Geometry check sheet. Reference: the model listing, model coordinates, mm. Round coordinates to 2 decimals unless told otherwise and drop trailing zeros. Write each loop counter-clockwise with the first axis right and the second up, starting at its lowest first coordinate (ties: lowest second). Pieces come first, ordered by that corner, then holes. Notation, with made-up numbers: (-11, 17) -> (20, 17) arc R25 ccw to (20, 39) -> close; hole circle Ø11 at (10, 76.25). An arc over 180 degrees is marked (long way). Put each result on its own line as item: value. Start each with the question number.
from build123d import *

# Parameters (mm, degrees)
SKETCH1_W           = 135
SKETCH1_H           = 75
BOSS_EXTRUDE1_DEPTH = 2.5
CUT_EXTRUDE1_REACH  = 4.5
SKETCH2_R           = 1.7


with BuildPart() as part:
    # Sketch1 → Boss-Extrude1 (new body)
    with BuildSketch(Plane(origin=(0, 0, 0), x_dir=(1, 0, 0), z_dir=(0, 1, 0))):
        Rectangle(SKETCH1_W, SKETCH1_H)
    extrude(amount=BOSS_EXTRUDE1_DEPTH)

    # Sketch2 → Cut-Extrude1 (cut, up to next)
    with BuildSketch(Plane(origin=(0, 0, 0), x_dir=(1, 0, 0), z_dir=(0, 1, 0)), mode=Mode.PRIVATE) as cut_extrude1_sk1:
        with Locations((63.75, -34)):
            Circle(SKETCH2_R)
    cut_extrude1_tool1 = extrude(cut_extrude1_sk1.sketch, amount=CUT_EXTRUDE1_REACH, mode=Mode.PRIVATE) & part.part
    add(cut_extrude1_tool1.solids().sort_by_distance((63.75, 0, 34))[0], mode=Mode.SUBTRACT)
    # Sketch2 → Cut-Extrude1 (cut, up to next)
    with BuildSketch(Plane(origin=(0, 0, 0), x_dir=(1, 0, 0), z_dir=(0, 1, 0)), mode=Mode.PRIVATE) as cut_extrude1_sk2:
        with Locations((63.75, 2)):
            Circle(SKETCH2_R)
    cut_extrude1_tool2 = extrude(cut_extrude1_sk2.sketch, amount=CUT_EXTRUDE1_REACH, mode=Mode.PRIVATE) & part.part
    add(cut_extrude1_tool2.solids().sort_by_distance((63.75, 0, -2))[0], mode=Mode.SUBTRACT)
    # Sketch2 → Cut-Extrude1 (cut, up to next)
    with BuildSketch(Plane(origin=(0, 0, 0), x_dir=(1, 0, 0), z_dir=(0, 1, 0)), mode=Mode.PRIVATE) as cut_extrude1_sk3:
        with Locations((-63.75, -34)):
            Circle(SKETCH2_R)
    cut_extrude1_tool3 = extrude(cut_extrude1_sk3.sketch, amount=CUT_EXTRUDE1_REACH, mode=Mode.PRIVATE) & part.part
    add(cut_extrude1_tool3.solids().sort_by_distance((-63.75, 0, 34))[0], mode=Mode.SUBTRACT)
    # Sketch2 → Cut-Extrude1 (cut, up to next)
    with BuildSketch(Plane(origin=(0, 0, 0), x_dir=(1, 0, 0), z_dir=(0, 1, 0)), mode=Mode.PRIVATE) as cut_extrude1_sk4:
        with Locations((-63.75, 34)):
            Circle(SKETCH2_R)
    cut_extrude1_tool4 = extrude(cut_extrude1_sk4.sketch, amount=CUT_EXTRUDE1_REACH, mode=Mode.PRIVATE) & part.part
    add(cut_extrude1_tool4.solids().sort_by_distance((-63.75, 0, -34))[0], mode=Mode.SUBTRACT)


solid = part.part
(1) Mould release check, pull along X, two halves, no side actions. Record for faces 1 (the cylindrical face through (62.4, 1.23, 35.03)), 2 (the flat face through (-1, 0, -1)), 3 (the flat face through (67.5, 1, 1)): +X half, -X half, draft (parallel to the pull), parting line (faces both ways), or undercut.
(2) Sectioned sample at B-B (z = 34). Record the cut outline in (x, y).
(3) Sectioned sample at C-C (z = -34). Record the cut outline in (x, y), and give its area (3 significant figures).
(4) Go/stop test with a flat-tipped pin: pin 1 Ø2 at (x, z) = (-63.75, 34) entering from +Y. Record where the tip stops, or that it passes through.
(5) Sectioned sample at A-A (x = -63.75). Record the cut outline in (y, z), and give its area (4 significant figures).
(6) Material ranges on L1, parallel to Z at x = -63.75, y = 1; L2, parallel to X at y = 1.8, z = 34; L3, parallel to X at y = 1.8, z = -2, recorded low to high. Write a range as from..to.
Found:
1. face 1: undercut
1. face 2: draft
1. face 3: +X half
2. outline: (-67.5, 0) -> (-65.45, 0) -> (-65.45, 2.5) -> (-67.5, 2.5) -> close; (-62.05, 0) -> (62.05, 0) -> (62.05, 2.5) -> (-62.05, 2.5) -> close; (65.45, 0) -> (67.5, 0) -> (67.5, 2.5) -> (65.45, 2.5) -> close
3. outline: (-67.5, 0) -> (-65.45, 0) -> (-65.45, 2.5) -> (-67.5, 2.5) -> close; (-62.05, 0) -> (67.5, 0) -> (67.5, 2.5) -> (-62.05, 2.5) -> close
3. area: 329 mm2
4. pin 1: through
5. outline: (0, -37.5) -> (2.5, -37.5) -> (2.5, -35.7) -> (0, -35.7) -> close; (0, -32.3) -> (2.5, -32.3) -> (2.5, 32.3) -> (0, 32.3) -> close; (0, 35.7) -> (2.5, 35.7) -> (2.5, 37.5) -> (0, 37.5) -> close
5. area: 170.5 mm2
6. L1: -37.5..-35.7, -32.3..32.3, 35.7..37.5
6. L2: -67.5..-65.45, -62.05..62.05, 65.45..67.5
6. L3: -67.5..62.05, 65.45..67.5
